Geometry: final body of the model. Coordinates: model frame, mm. A direction names the side the tool comes from. Give positions to 0.01 mm unless a question says otherwise; leave off trailing zeros. Order: outer loops, then holes, each group sorted by start corner. A loop starts at its lowest first (then second) coordinate and runs counter-clockwise, first axis right, second up. Notation, with made-up numbers: (-10, -39) - (45, -39) arc R31 cw to (45, -10) - close; hole circle Ø4 at (8, -32.75). An arc over 180 degrees is marked (long way). Put each result on its own line as item: value. Start each with the question number.
1. First-contact query: P1, Ø3, axis at x = -9.5, z = 16.5, coming from the +Y side; P2, Ø5, axis at x = -20, z = 31.5, coming from the +Y side; P3, Ø3, axis at x = 10, z = 30, coming from the -Y side. Flat tips, straight axial feed; report the tip coordinate or a pass-through.
2. Mould query, pull axis Y, two halves, no side actions, for faces 1 (the flat face through (7.5, -12, 20)), 2 (the cylindrical face through (-21.513, 12.735, 19.72)), 3 (the flat face through (5, 0, 0)). Classes: pulls with the +Y half, pulls with the -Y half, needs draft (parallel to the pull), parting line crosses it, or undercut.
3. Section B-B on y = 19. Return the cut outline in (x, z).
4. Section D-D on z = 31.5. Return the cut outline in (x, y), plus the area to 3 significant figures.
5. Section C-C on x = -16. Return the cut outline in (y, z), plus the area to 3 significant figures.
6. Ray query, line 1 along X through (y, z) = (2, 13); line 2 along X through (y, z) = (-0.5, 31) (3 decimals); line 3 along Y through (x, z) = (-15.5, 22). Return the intervals inside material, ascending. Write a range as from..to.
7. Set-up query: faces 4 (the flat face through (-14.38, -0.36, 19.72)), 5 (the cylindrical face through (21.785, 12.264, 19.72)). Return all of +Z, -Z, +X, -X, +Y, -Y with unobstructed straight access to the full face (end or side cutting, diameter ignored); none if empty.
8. Section A-A on y = 0. Return the cut outline in (x, z), plus the area to 3 significant figures.
from build123d import *

# Parameters (mm, degrees)
SKETCH1_R           = 2.5
BOSS_EXTRUDE1_DEPTH = 40


with BuildPart() as part:
    # Sketch1 → Boss-Extrude1 (new body)
    # profile 1 of 7: a face of its own
    with BuildSketch(Plane.XY):
        with BuildLine():
            Line((-7.5, -4.330127019), (-7.5, 0))
            ThreePointArc((-7.5, 0), (-6.495190528, 3.75), (-3.75, 6.495190528))
            Line((-3.75, 6.495190528), (0, 8.660254038))
            Line((0, 8.660254038), (-13.570508076, 16.495190528))
            ThreePointArc((-13.570508076, 16.495190528), (-10.967861495, 21.068660914), (-6.663448066, 24.095610801))
            ThreePointArc((-6.663448066, 24.095610801), (-21.650635095, 12.5), (-24.199135106, -6.277090099))
            ThreePointArc((-24.199135106, -6.277090099), (-23.729926323, -1.035883777), (-21.070508076, 3.504809472))
            Line((-21.070508076, 3.504809472), (-7.5, -4.330127019))
        make_face()
    # profile 2 of 7: a face of its own
    with BuildSketch(Plane.XY):
        with BuildLine():
            Line((13.570508076, 16.495190528), (0, 8.660254038))
            Line((0, 8.660254038), (3.75, 6.495190528))
            ThreePointArc((3.75, 6.495190528), (6.495190528, 3.75), (7.5, 0))
            Line((7.5, 0), (7.5, -4.330127019))
            Line((7.5, -4.330127019), (21.070508076, 3.504809472))
            ThreePointArc((21.070508076, 3.504809472), (23.729926323, -1.035883777), (24.199135106, -6.277090099))
            ThreePointArc((24.199135106, -6.277090099), (21.650635095, 12.5), (6.663448066, 24.095610801))
            ThreePointArc((6.663448066, 24.095610801), (10.967861495, 21.068660914), (13.570508076, 16.495190528))
        make_face()
    # profile 3 of 7: a face of its own
    with BuildSketch(Plane.XY):
        with BuildLine():
            Line((-3.75, -6.495190528), (-7.5, -4.330127019))
            Line((-7.5, -4.330127019), (-7.5, -20))
            ThreePointArc((-7.5, -20), (-12.762064828, -20.032777137), (-17.53568704, -17.818520702))
            ThreePointArc((-17.53568704, -17.818520702), (0, -25), (17.53568704, -17.818520702))
            ThreePointArc((17.53568704, -17.818520702), (12.762064828, -20.032777137), (7.5, -20))
            Line((7.5, -20), (7.5, -4.330127019))
            Line((7.5, -4.330127019), (3.75, -6.495190528))
            ThreePointArc((3.75, -6.495190528), (0, -7.5), (-3.75, -6.495190528))
        make_face()
    # profile 4 of 7: a face of its own
    with BuildSketch(Plane.XY):
        with BuildLine():
            Line((0, 8.660254038), (-3.75, 6.495190528))
            ThreePointArc((-3.75, 6.495190528), (0, 7.5), (3.75, 6.495190528))
            Line((3.75, 6.495190528), (0, 8.660254038))
        make_face()
    # profile 5 of 7: a face of its own
    with BuildSketch(Plane.XY):
        with BuildLine():
            ThreePointArc((-3.75, -6.495190528), (-6.495190528, -3.75), (-7.5, 0))
            Line((-7.5, 0), (-7.5, -4.330127019))
            Line((-7.5, -4.330127019), (-3.75, -6.495190528))
        make_face()
    # profile 6 of 7: a face of its own
    with BuildSketch(Plane.XY):
        with BuildLine():
            ThreePointArc((7.5, 0), (6.495190528, -3.75), (3.75, -6.495190528))
            Line((3.75, -6.495190528), (7.5, -4.330127019))
            Line((7.5, -4.330127019), (7.5, 0))
        make_face()
    # profile 7 of 7: a face of its own
    with BuildSketch(Plane.XY):
        with BuildLine():
            ThreePointArc((-3.75, 6.495190528), (-6.495190528, 3.75), (-7.5, 0))
            ThreePointArc((-7.5, 0), (-6.495190528, -3.75), (-3.75, -6.495190528))
            ThreePointArc((-3.75, -6.495190528), (0, -7.5), (3.75, -6.495190528))
            ThreePointArc((3.75, -6.495190528), (6.495190528, -3.75), (7.5, 0))
            ThreePointArc((7.5, 0), (6.495190528, 3.75), (3.75, 6.495190528))
            ThreePointArc((3.75, 6.495190528), (0, 7.5), (-3.75, 6.495190528))
        make_face()
        Circle(SKETCH1_R, mode=Mode.SUBTRACT)
    extrude(amount=BOSS_EXTRUDE1_DEPTH)


solid = part.part
Resolved:
1. P1: y = 23.69
1. P2: y = 17.85
1. P3: y = -23.51
2. face 1: undercut
2. face 2: parting line crosses it
2. face 3: needs draft
3. outline: (-16.25, 0) - (-12.48, 0) - (-12.48, 40) - (-16.25, 40) - close; (12.48, 0) - (16.25, 0) - (16.25, 40) - (12.48, 40) - close
4. outline: (-24.2, -6.28) arc R12.04 cw to (-21.07, 3.5) - (-7.5, -4.33) - (-7.5, -20) arc R12.04 cw to (-17.54, -17.82) arc R25 ccw to (17.54, -17.82) arc R12.04 cw to (7.5, -20) - (7.5, -4.33) - (21.07, 3.5) arc R12.04 cw to (24.2, -6.28) arc R25 ccw to (6.66, 24.1) arc R12.04 cw to (13.57, 16.5) - (0, 8.66) - (-13.57, 16.5) arc R12.04 cw to (-6.66, 24.1) arc R25 ccw to start; hole circle Ø5 at (0, 0)
4. area: 1,090 mm^2
5. outline: (-19.21, 0) - (-18.82, 0) - (-18.82, 40) - (-19.21, 40) - close; (0.58, 0) - (19.21, 0) - (19.21, 40) - (0.58, 40) - close
5. area: 761 mm^2
6. line 1: -24.92..-22.26, -18.46..-1.5, 1.5..18.46, 22.26..24.92
6. line 2: -24.995..-23.545, -14.134..-2.449, 2.449..14.134, 23.545..24.995
6. line 3: -19.62..-19.08, 0.29..19.62
7. face 4: +Z, -Z
7. face 5: +Z, -Z, +X
8. outline: (-25, 0) - (-23.35, 0) - (-23.35, 40) - (-25, 40) - close; (-15, 0) - (-2.5, 0) - (-2.5, 40) - (-15, 40) - close; (2.5, 0) - (15, 0) - (15, 40) - (2.5, 40) - close; (23.35, 0) - (25, 0) - (25, 40) - (23.35, 40) - close
8. area: 1,130 mm^2
